Drawing for the job (mm, zero at the part's lowest x, y, z). Coordinates: 2 decimals unless noted, no trailing zeros. Write each loop counter-clockwise with the first axis right and the second up, starting at its lowest first coordinate (ties: lowest second). Pieces come first, ordered by that corner, then holes. Notation, with made-up numbers: (-36, 2.5) -> (-9, 2.5) arc R19 cw to (-9, 16.5) -> close; hole circle Ø10 at (45.25, 27). An arc over 180 degrees is marked (long way). Write item = value, one per line. Start each with the question number.
Q1. Band-saw the part on B-B, the plane z = 91. List the corners of the cut face in (x, y).
Q2. Probe line 1 (Z direction, x = 4, y = 0.85); line 2 (X direction, y = 0.5, z = 91). List the from-to ranges inside material, lowest first.
Q3. Band-saw the part on A-A, the plane x = 142.5. List the corners of the cut face in (y, z), plus the area to 3 significant figures.
Q4. Pin check, flat tip, straight feed: P1, Ø2, axis at x = 4, z = 91, coming from the -Y side. Stop position of the tip, or through.
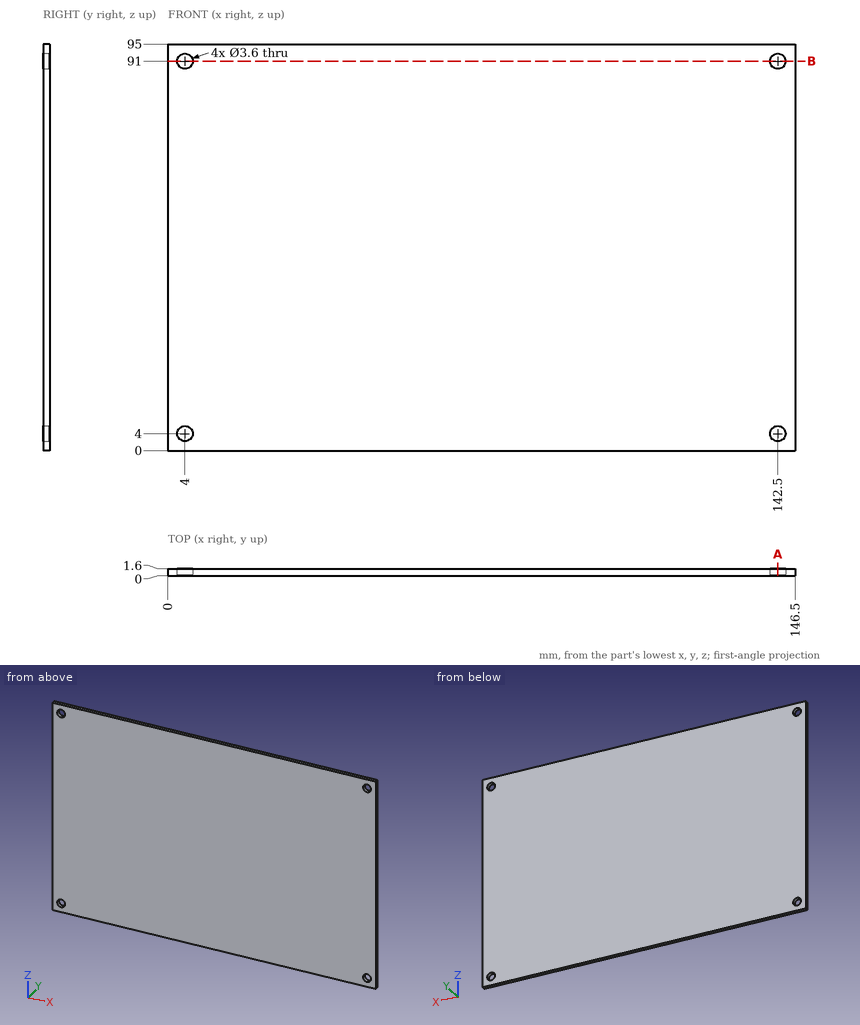
Ans:
q1.outline = (0, 0) -> (2.2, 0) -> (2.2, 1.6) -> (0, 1.6) -> close; (5.8, 0) -> (140.7, 0) -> (140.7, 1.6) -> (5.8, 1.6) -> close; (144.3, 0) -> (146.5, 0) -> (146.5, 1.6) -> (144.3, 1.6) -> close
q2.line_1 = 0 to 2.2, 5.8 to 89.2, 92.8 to 95
q2.line_2 = 0 to 2.2, 5.8 to 140.7, 144.3 to 146.5
q3.outline = (0, 0) -> (1.6, 0) -> (1.6, 2.2) -> (0, 2.2) -> close; (0, 5.8) -> (1.6, 5.8) -> (1.6, 89.2) -> (0, 89.2) -> close; (0, 92.8) -> (1.6, 92.8) -> (1.6, 95) -> (0, 95) -> close
q3.area = 140 mm2
q4.P1 = through
